Autodesk Inventor part; units mm, degrees
ref_plane "YZ Plane" through (0, 0, 0) normal (1, 0, 0) x (0, 1, 0)
ref_plane "XZ Plane" through (0, 0, 0) normal (0, 1, 0) x (-1, 0, 0)
ref_plane "XY Plane" through (0, 0, 0) normal (0, 0, 1) x (1, 0, 0)
sketch "Sketch1" plane through (0, 0, 0) normal (0, 0, 1) x (1, 0, 0)
  line L0 (-4.8449, 2.8898) -> (4.6751, 2.8898)
  line L1 (4.6751, 2.8898) -> (4.6751, -5.0302)
  line L2 (4.6751, -5.0302) -> (-4.8449, -5.0302)
  line L3 (-4.8449, -5.0302) -> (-4.8449, 2.8898)
  point P0 (0, 0)
  dimension "d0" = 9.52
  dimension "d1" = 7.92
extrude "Extrusion1" add sketch "Sketch1" along normal blind 1.65
sketch "Sketch2" plane through (4.6751, -5.0302, 0) normal (1, 0, 0) x (0, 0, -1)
  line L0 (-1.65, 0) -> (-1.65, 7.92)
  line L1 (-1.65, 3.84) -> (-6.4, 3.84)
  line L2 (-6.4, 3.84) -> (-6.4, 4.86)
  line L3 (-6.4, 4.86) -> (-1.65, 4.86)
  line L4 (-1.65, 4.86) -> (-1.65, 3.84)
  line L5 (-1.65, 0) -> (-6.4, 0)
  line L6 (-6.4, 0) -> (-6.4, 2.11)
  line L7 (-6.4, 2.11) -> (-1.65, 2.11)
  line L8 (-1.65, 2.11) -> (-1.65, 0)
  point P0 (0, 5.0302)
  dimension "d4" = 1.73
  dimension "d5" = 2.11
  dimension "d6" = 1.02
  dimension "d7" = 4.75
  dimension "d8" = 4.75
extrude "Extrusion2" add sketch "Sketch2" against normal blind 9.53
sketch "Sketch3" plane through (0, 0, 0) normal (0, 0, -1) x (-1, 0, 0)
  circle A0 centre (0.0849, -1.0702) radius 3
  point P0 (0, 0)
  dimension "d11" = 6
extrude "Extrusion3" add sketch "Sketch3" along normal blind 11.03
ref_plane "Work Plane1" through (-0.0849, -1.0702, -7.36) normal (0, 0, -1) x (-1, 0, 0)
sketch "Sketch4" plane through (-0.0849, -1.0702, -7.36) normal (0, 0, -1) x (-1, 0, 0)
  line L0 (4.4515, 0.275) -> (2.3983, -3.725)
  line L1 (2.3983, -3.725) -> (-2.0924, -3.9469)
  line L2 (-2.0924, -3.9469) -> (-4.5299, -0.1688)
  line L3 (-4.5299, -0.1688) -> (-2.4767, 3.8312)
  line L4 (-2.4767, 3.8312) -> (2.014, 4.0531)
  line L5 (2.014, 4.0531) -> (4.4515, 0.275)
  point P0 (-0.0849, 1.0702)
  point P1 (-0.0392, 0.0531)
  dimension "d15" = 4
extrude "Extrusion4" add sketch "Sketch4" against normal blind 3.67
sketch "Sketch5" plane through (-0.0849, -1.0702, -11.03) normal (0, 0, -1) x (-1, 0, 0)
  circle A0 centre (0, 0) radius 3
  circle A1 centre (0, 0) radius 2.3707
  point P0 (-0.0849, 1.0702)
extrude "Extrusion5" cut sketch "Sketch5" against normal blind 3.67 contours A1
properties part number "SMA_EdgeMale"
Source: CAD feature listing. Evaluate the final solid. Frame: model axes, mm. A direction names the side the tool comes from. Round coordinates to 2 decimals unless told otherwise and drop trailing zeros. Loops run counter-clockwise (first coordinate to the right, second up) from the corner with the lowest first, then second, coordinate; pieces in that order, holes last.
(1) Material intervals for probe 1 along Z at (x, y) = (-3, 0); probe 2 along Y at (x, z) = (4.25, 3); probe 3 along Z at (x, y) = (4.25, -0.25), sorted ascending.
From the geometry:
probe 1: z = -7.36 to -3.69, 0 to 1.65
probe 2: y = -5.03 to -2.92, -1.19 to -0.17
probe 3: z = 0 to 6.4
(2) Section query B-B (x = 3.5). Output: boundary loops of the cut face in (y, z).
From the geometry:
outline: (-5.03, 0) - (2.89, 0) - (2.89, 1.65) - (-0.17, 1.65) - (-0.17, 6.4) - (-1.19, 6.4) - (-1.19, 1.65) - (-2.92, 1.65) - (-2.92, 6.4) - (-5.03, 6.4) - close; (-2.7, -7.36) - (0.6, -7.36) - (0.6, -3.69) - (-2.7, -3.69) - close
(3) Pull-direction query (Z, two-part tool) for faces 1 (the flat face through (-3.3, 1.12, -5.55)), 2 (the flat face through (3, -2, -3.69)), 3 (the flat face through (0, -2, 1.65)); classes: +Z half, -Z half, draft (parallel to the pull), parting line (faces both ways), or undercut.
From the geometry:
face 1: draft
face 2: undercut
face 3: +Z half
(4) Contact query for flat-ended pins moving along their axis: pin 1 Ø5 at (x, z) = (-0.5, 4.5) entering from +Y; pin 2 Ø0.5 at (x, y) = (2, -1.5) entering from +Z; pin 3 Ø1.5 at (x, z) = (1, -3.5) entering from -Y. Output: stop coordinate, or through.
From the geometry:
pin 1: stops at y = -0.17
pin 2: stops at z = 1.65
pin 3: stops at y = -5
(5) Section query D-D (x = -1.5). Output: boundary loops of the cut face in (y, z), and give its area (3 significant figures).
From the geometry:
outline: (-5.03, 0) - (-3.72, 0) - (-3.72, -3.69) - (-4.84, -3.69) - (-4.84, -7.36) - (-3.72, -7.36) - (-3.72, -11.03) - (-2.97, -11.03) - (-2.97, -7.36) - (0.83, -7.36) - (0.83, -11.03) - (1.58, -11.03) - (1.58, -7.36) - (2.95, -7.36) - (2.95, -3.69) - (1.58, -3.69) - (1.58, 0) - (2.89, 0) - (2.89, 1.65) - (-0.17, 1.65) - (-0.17, 6.4) - (-1.19, 6.4) - (-1.19, 1.65) - (-2.92, 1.65) - (-2.92, 6.4) - (-5.03, 6.4) - close
area: 81.5 mm2
(6) Section query A-A (z = 5.25). Output: boundary loops of the cut face in (x, y).
From the geometry:
outline: (-4.85, -5.03) - (4.68, -5.03) - (4.68, -2.92) - (-4.85, -2.92) - close; (-4.85, -1.19) - (4.68, -1.19) - (4.68, -0.17) - (-4.85, -0.17) - close
(7) Access query for faces 4 (the flat face through (0, -1, -7.36)), 5 (the flat face through (0, -0.17, 4)), 6 (the flat face through (3.433, 0.733, -5.551)), 7 (the flat face through (-0.269, -4.905, -5.551)), 8 (the flat face through (0, -1.19, 4)). Directions: +Z, -Z, +X, -X, +Y, -Y. A direction counts if a zero-diameter tool reaches every point of the face in a straight line with its end or side. Return the directions, or none.
From the geometry:
face 4: -Z
face 5: +Z, +X, -X, +Y
face 6: -Z, +X, +Y
face 7: -Z, -X, -Y
face 8: +Z, +X, -X
